Read the model definition and answer for the solid it produces. Units are mm, in the model's axes. A direction names the side the tool comes from. Coordinates: 2 decimals unless noted, no trailing zeros. Loops run counter-clockwise (first coordinate to the right, second up) from the corner with the lowest first, then second, coordinate; pieces in that order, holes last. Notation, with made-up numbers: (-13.5, -33.5) -> (36.5, -33.5) arc R18 cw to (36.5, -5.5) -> close; hole circle Ø4 at (-29, 38.25). An arc over 180 degrees is marked (long way). Answer as a JSON object with one key per item and string values. Group by question number.
Q1. Straight lines are drawn through the part: line 1 along Y through (x, z) = (3.75, -4.25); line 2 along Y through (x, z) = (7, -4.75). For each, find the intervals that lie inside material, in ascending order. Write a range as [from, to].
Q2. Determine the mould class of faces 3 (the cylindrical face through (3.7, -0.75, -6.59)), 4 (the flat face through (4, -2, -10)), 5 (the flat face through (4, -3, -5)) for opening direction Z: released by +Z, released by -Z, zero draft, split by the parting line, or undercut.
Q3. The part is cut by section B-B on z = -0.5. Write down the section's boundary in (x, y), and give its area (3 significant figures).
Q4. For faces 1 (the cylindrical face through (3.7, -0.75, -8.59)), 2 (the flat face through (3.9, 0, -1.6)), determine the directions among +Z, -Z, +X, -X, +Y, -Y from which every point of the face is accessible in a straight line to the end or side of a thin tool.
from build123d import *

# Parameters (mm, degrees)
SKETCH2_W           = 10
SKETCH2_H           = 3
BOSS_EXTRUDE1_DEPTH = 7.5
CUT_EXTRUDE2_DEPTH  = 13.854960132
LPATTERN2_COUNT     = 10
LPATTERN2_PITCH     = 2
FILLET2_START       = -1
FILLET2_DEPTH       = 9
SKETCH3_W           = 10
SKETCH3_H           = 3
BOSS_EXTRUDE2_DEPTH = 6


with BuildPart() as part:
    # Sketch2 → Boss-Extrude1 (new body)
    with BuildSketch(Plane(origin=(0, 0, 0), x_dir=(0, 0, -1), z_dir=(1, 0, 0))):
        with Locations((5, -1.5)):
            Rectangle(SKETCH2_W, SKETCH2_H)
    extrude(amount=BOSS_EXTRUDE1_DEPTH)

    # Sketch1 → Cut-Extrude2 (cut, through all)
    with BuildSketch(Plane(origin=(0, 0, 0), x_dir=(0, 0, -1), z_dir=(1, 0, 0))):
        with BuildLine():
            ThreePointArc((0.10112359, -0.438202237), (0.045620517, -0.221237163), (0.080384758, 0))
            Line((0.080384758, 0), (0, 0))
            ThreePointArc((0, 0), (0.025608803, -0.224859501), (0.10112359, -0.438202237))
        make_face()
        with BuildLine():
            ThreePointArc((1.155, -0.195), (1.146082164, -0.095907769), (1.119615242, 0))
            Line((1.119615242, 0), (0.080384758, 0))
            ThreePointArc((0.080384758, 0), (0.045620517, -0.221237163), (0.10112359, -0.438202237))
            ThreePointArc((0.10112359, -0.438202237), (0.6, -0.75), (1.09887641, -0.438202237))
            ThreePointArc((1.09887641, -0.438202237), (1.140787115, -0.319797021), (1.155, -0.195))
        make_face()
        with BuildLine():
            Line((0.080384758, 0), (1.119615242, 0))
            ThreePointArc((1.119615242, 0), (0.6, 0.36), (0.080384758, 0))
        make_face()
        with BuildLine():
            ThreePointArc((1.09887641, -0.438202237), (1.174391197, -0.224859501), (1.2, 0))
            Line((1.2, 0), (1.119615242, 0))
            ThreePointArc((1.119615242, 0), (1.146082164, -0.095907769), (1.155, -0.195))
            ThreePointArc((1.155, -0.195), (1.140787115, -0.319797021), (1.09887641, -0.438202237))
        make_face()
    cut_extrude2 = extrude(amount=CUT_EXTRUDE2_DEPTH, mode=Mode.SUBTRACT)

    # LPattern2: Cut-Extrude2 ×10
    with Locations(*[(0, 0, -i * LPATTERN2_PITCH) for i in range(1, LPATTERN2_COUNT)]):
        add(cut_extrude2, mode=Mode.SUBTRACT)

    # Fillet2: read off the stored shape, not the designer's step
    # Fillet2 outline → Fillet2 (cut)
    with BuildSketch(Plane.YZ.offset(FILLET2_START)):
        with BuildLine():
            Line((0, -10), (0, -9.85))
            ThreePointArc((0, -9.85), (-0.043933983, -9.956066017), (-0.15, -10))
            Line((-0.15, -10), (0, -10))
        make_face()
        with BuildLine():
            ThreePointArc((-0.130434783, -9.191456891), (-0.037228588, -9.241268354), (0, -9.340175425))
            Line((0, -9.340175425), (0, -9.2))
            ThreePointArc((0, -9.2), (-0.065357129, -9.197861937), (-0.130434783, -9.191456891))
        make_face()
        with BuildLine():
            Line((0, -8), (0, -7.859824575))
            ThreePointArc((0, -7.859824575), (-0.037228588, -7.958731646), (-0.130434783, -8.008543109))
            ThreePointArc((-0.130434783, -8.008543109), (-0.065357129, -8.002138063), (0, -8))
        make_face()
        with BuildLine():
            ThreePointArc((-0.130434783, -7.191456891), (-0.037228588, -7.241268354), (0, -7.340175425))
            Line((0, -7.340175425), (0, -7.2))
            ThreePointArc((0, -7.2), (-0.065357129, -7.197861937), (-0.130434783, -7.191456891))
        make_face()
        with BuildLine():
            Line((0, -6), (0, -5.859824575))
            ThreePointArc((0, -5.859824575), (-0.037228588, -5.958731646), (-0.130434783, -6.008543109))
            ThreePointArc((-0.130434783, -6.008543109), (-0.065357129, -6.002138063), (0, -6))
        make_face()
        with BuildLine():
            ThreePointArc((-0.130434783, -5.191456891), (-0.037228588, -5.241268354), (0, -5.340175425))
            Line((0, -5.340175425), (0, -5.2))
            ThreePointArc((0, -5.2), (-0.065357129, -5.197861937), (-0.130434783, -5.191456891))
        make_face()
        with BuildLine():
            Line((0, -4), (0, -3.859824575))
            ThreePointArc((0, -3.859824575), (-0.037228588, -3.958731646), (-0.130434783, -4.008543109))
            ThreePointArc((-0.130434783, -4.008543109), (-0.065357129, -4.002138063), (0, -4))
        make_face()
        with BuildLine():
            ThreePointArc((-0.130434783, -3.191456891), (-0.037228588, -3.241268354), (0, -3.340175425))
            Line((0, -3.340175425), (0, -3.2))
            ThreePointArc((0, -3.2), (-0.065357129, -3.197861937), (-0.130434783, -3.191456891))
        make_face()
        with BuildLine():
            Line((0, -2), (0, -1.859824575))
            ThreePointArc((0, -1.859824575), (-0.037228588, -1.958731646), (-0.130434783, -2.008543109))
            ThreePointArc((-0.130434783, -2.008543109), (-0.065357129, -2.002138063), (0, -2))
        make_face()
        with BuildLine():
            ThreePointArc((-0.737701575, 0), (-0.601941305, -0.086210119), (-0.622233155, -0.245744681))
            ThreePointArc((-0.622233155, -0.245744681), (-0.537928158, -0.163622551), (-0.438202247, -0.101123596))
            ThreePointArc((-0.438202247, -0.101123596), (-0.224859507, -0.025608804), (0, 0))
            Line((0, 0), (-0.737701575, 0))
        make_face()
        with BuildLine():
            ThreePointArc((-0.130434783, -1.191456891), (-0.037228588, -1.241268354), (0, -1.340175425))
            Line((0, -1.340175425), (0, -1.2))
            ThreePointArc((0, -1.2), (-0.065357129, -1.197861937), (-0.130434783, -1.191456891))
        make_face()
    extrude(amount=FILLET2_DEPTH, mode=Mode.SUBTRACT)

    # Sketch3 → Boss-Extrude2 (add)
    with BuildSketch(Plane(origin=(7.5, 0, 0), x_dir=(0, 0, -1), z_dir=(1, 0, 0))):
        with Locations((5, -1.5)):
            Rectangle(SKETCH3_W, SKETCH3_H)
    boss_extrude2 = extrude(amount=BOSS_EXTRUDE2_DEPTH)

    # Mirror1: Boss-Extrude2 across plane
    add(boss_extrude2.mirror(Plane.ZY.offset(-3.75)))


solid = part.part
Final values:
{
 "1": {"line 1": "y = [-3, -0.63]", "line 2": "y = [-3, -0.73]"},
 "2": {"face 3": "undercut", "face 4": "released by -Z", "face 5": "zero draft"},
 "3": {"outline": "(-6, -3) -> (13.5, -3) -> (13.5, 0) -> (7.5, 0) -> (7.5, -0.74) -> (0, -0.74) -> (0, 0) -> (-6, 0) -> close", "area": "52.9 mm2"},
 "4": {"face 1": "+Y", "face 2": "+Z, -Z, +X, -X, +Y"}
}
